For this review, use the dimensioned drawing (mm, ordinates from the lowest corner) and the shaded views. Coordinates: 2 decimals unless noted, no trailing zeros. Loops run counter-clockwise (first coordinate to the right, second up) from the corner with the lowest first, then second, coordinate; pieces in that order, holes last. Notation, with made-up numbers: M -31.5,-12 L -10.5,-12 A8 ccw -10.5,0 Z; hole C -18.5,9 d10. An arc over 180 degrees is marked long. Write item = value, one per line.
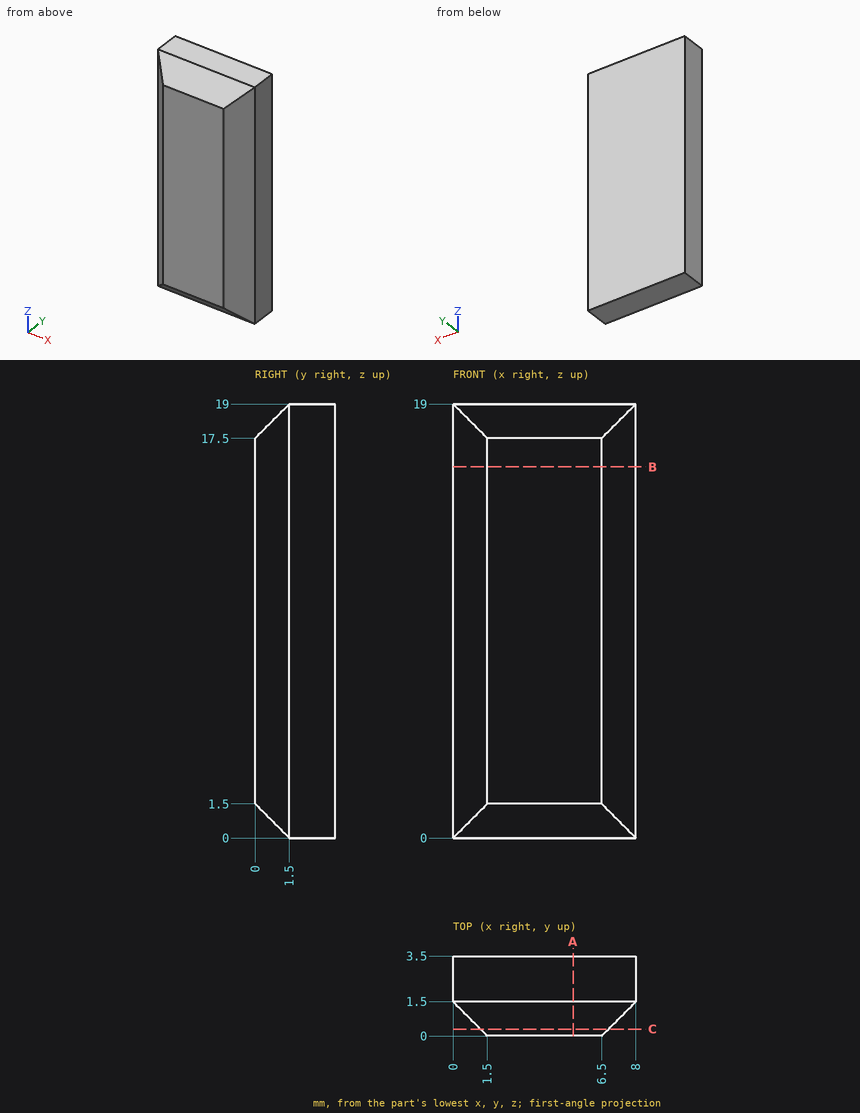
Q1. Add section A-A (x = 5.25). Write out the cut boundary in (y, z).
Solved:
outline = M 0,1.5 L 1.5,0 L 3.5,0 L 3.5,19 L 1.5,19 L 0,17.5 Z
Q2. For line 1 along X through (y, z) = (0.85, 9); line 2 along Y through (x, z) = (6.75, 4.75); line 3 along Z through (x, y) = (2.75, 0.4), list the stretches that pass through material, from the lowest coordinate up.
Solved:
line_1 = 0.65 to 7.35
line_2 = 0.25 to 3.5
line_3 = 1.1 to 17.9
Q3. Add section C-C (y = 0.3). Write out the cut boundary in (x, z), and give its area (3 significant figures).
Solved:
outline = M 1.2,1.2 L 6.8,1.2 L 6.8,17.8 L 1.2,17.8 Z
area = 93.0 mm²
Q4. Add section B-B (z = 16.25). Write out the cut boundary in (x, y).
Solved:
outline = M 0,1.5 L 1.5,0 L 6.5,0 L 8,1.5 L 8,3.5 L 0,3.5 Z
